Work out the finished part from the listing and answer in its coordinate system (mm). Give positions to 0.01 mm unless a question says otherwise; leave off trailing zeros. Loops run counter-clockwise (first coordinate to the right, second up) from the corner with the lowest first, then second, coordinate; pieces in that order, holes last.
from build123d import *

# Parameters (mm, degrees)
F0_W      = 22
F0_H      = 615
F1_DEPTH  = 20
F2_W      = 12
F2_H      = 20
F3_DEPTH  = 25
F4_W      = 12
F4_H      = 20
F5_DEPTH  = 30
F6_R      = 9.99999
F7_R      = 2.5
F8_DEPTH  = 30
F10_DEPTH = 25
F11_R     = 1
F12_SIZE  = 3
F13_R     = 2


# Not quite as in the source:
# - a fillet or chamfer is up to 0.001 mm smaller than in the source, because OpenCascade refuses the exact size


with BuildPart() as f1:
    # F0 (on Front) → F1 (new body)
    with BuildSketch(Plane.XZ):
        Rectangle(F0_W, F0_H)
    extrude(amount=F1_DEPTH)

    # F2 (on face) → F3 (cut)
    with BuildSketch(Plane.XY.offset(307.5)):
        with Locations((0, -10)):
            Rectangle(F2_W, F2_H)
    extrude(amount=-F3_DEPTH, mode=Mode.SUBTRACT)

    # F4 (on face) → F5 (cut)
    with BuildSketch(Plane(origin=(0, 0, -307.5), x_dir=(1, 0, 0), z_dir=(0, 0, -1))):
        with Locations((0, 10)):
            Rectangle(F4_W, F4_H)
    extrude(amount=-F5_DEPTH, mode=Mode.SUBTRACT)

    # F6 (radius 10 in the source; OpenCascade refuses exactly that, so slightly less here)
    f6_edges = [f1.edges().sort_by_distance(p)[0] for p in [
        (-8.5, 0, -307.5),
        (8.5, 0, -307.5),
        (8.5, -20, -307.5),
        (-8.5, -20, -307.5),
        (-8.5, -20, 307.5),
        (-8.5, 0, 307.5),
        (8.5, 0, 307.5),
        (8.5, -20, 307.5),
    ]]
    fillet(f6_edges, radius=F6_R)

    # F7 (on face) → F8 (cut)
    with BuildSketch(Plane(origin=(-11, 0, 0), x_dir=(0, -1, 0), z_dir=(-1, 0, 0))):
        with Locations((10, 297.5)):
            Circle(F7_R)
        with Locations((10, -297.5)):
            Circle(F7_R)
    extrude(amount=-F8_DEPTH, mode=Mode.SUBTRACT)

    # F9 (on face) → F10 (cut)
    with BuildSketch(Plane.XZ.offset(20)):
        with BuildLine():
            ThreePointArc((6, 247.5), (0, 253.5), (-6, 247.5))
            Line((-6, 247.5), (-6, 117.5))
            ThreePointArc((-6, 117.5), (0, 111.5), (6, 117.5))
            Line((6, 117.5), (6, 247.5))
        make_face()
        with BuildLine():
            ThreePointArc((-6, -62.5), (0, -68.5), (6, -62.5))
            Line((6, -62.5), (6, 67.5))
            ThreePointArc((6, 67.5), (0, 73.5), (-6, 67.5))
            Line((-6, 67.5), (-6, -62.5))
        make_face()
        with BuildLine():
            Line((-6, -112.5), (-6, -242.5))
            ThreePointArc((-6, -242.5), (0, -248.5), (6, -242.5))
            Line((6, -242.5), (6, -112.5))
            ThreePointArc((6, -112.5), (0, -106.5), (-6, -112.5))
        make_face()
    extrude(amount=-F10_DEPTH, mode=Mode.SUBTRACT)

    # F11
    f11_edges = [f1.edges().sort_by_distance(p)[0] for p in [
        (11, 0, 0),
        (-11, 0, 0),
    ]]
    fillet(f11_edges, radius=F11_R)

    # F12
    f12_edges = [f1.edges().sort_by_distance(p)[0] for p in [
        (11, -7.5, 297.5),
        (11, -7.5, -297.5),
    ]]
    chamfer(f12_edges, length=F12_SIZE)

    # F13
    f13_edges = [f1.edges().sort_by_distance(p)[0] for p in [
        (-6, -10, -277.5),
        (6, -10, -277.5),
        (6, -10, 282.5),
        (-6, -10, 282.5),
    ]]
    fillet(f13_edges, radius=F13_R)


solid = f1.part
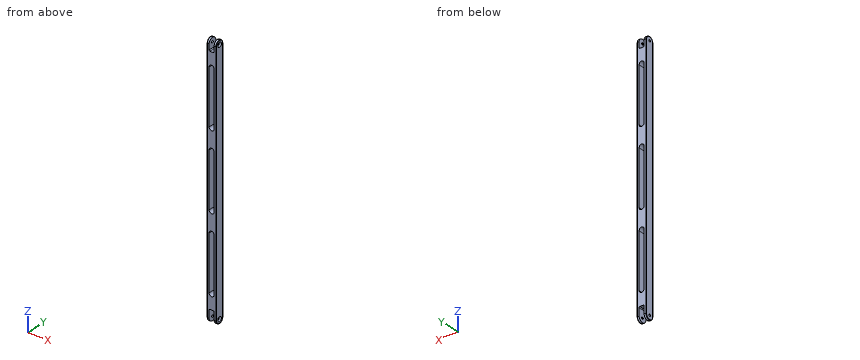
Item 1: Flat-ended cylindrical pins translate along their axes: pin 1 Ø1 at (x, y) = (7, -2.5) entering from -Z; pin 2 Ø5 at (x, z) = (2.5, 7.5) entering from -Y; pin 3 Ø6.5 at (y, z) = (-10, 297.5) entering from +X; pin 4 Ø6 at (y, z) = (-10, 297.5) entering from +X. Find the tip coordinate at first contact, or state that the pin passes through.
Item 2: Find section B-B, the plane x = 0. Write down the section's boundary in (y, z), plus the area to 3 significant figures.
Item 3: Find section A-A, the plane z = 167. Write down the section's boundary in (x, y), plus the area to 3 significant figures.
Item 4: Consider line 1 (Z direction, x = 0, y = -7.25); line 2 (X direction, y = -1.25, z = -43.5); line 3 (Y direction, x = -7.3, z = -297.5). Determine where each line is inside the solid, lowest interval first.
Ans:
1. pin 1: stops at z = -304.64
1. pin 2: passes through
1. pin 3: stops at x = 8.75
1. pin 4: stops at x = 8.5
2. outline: (-20, -277.5) - (0, -277.5) - (0, -248.5) - (-20, -248.5) - close; (-20, -106.5) - (0, -106.5) - (0, -68.5) - (-20, -68.5) - close; (-20, 73.5) - (0, 73.5) - (0, 111.5) - (-20, 111.5) - close; (-20, 253.5) - (0, 253.5) - (0, 282.5) - (-20, 282.5) - close
2. area: 2,680 mm2
3. outline: (-11, -19) arc R1 ccw to (-10, -20) - (-6, -20) - (-6, 0) - (-10, 0) arc R1 ccw to (-11, -1) - close; (6, -20) - (10, -20) arc R1 ccw to (11, -19) - (11, -1) arc R1 ccw to (10, 0) - (6, 0) - close
3. area: 199 mm2
4. line 1: z = -277.5 to -248.5, -106.5 to -68.5, 73.5 to 111.5, 253.5 to 282.5
4. line 2: x = -11 to -6, 6 to 11
4. line 3: y = -20 to -12.5, -7.5 to 0
